Model file for the job. Use its own axes, mm. Coordinates: 2 decimals unless noted, no trailing zeros. Write each loop counter-clockwise with the first axis right and the second up, starting at its lowest first coordinate (ties: lowest second). Pieces come first, ordered by that corner, then holes.
Q1. Drill centre lines: probe 1 along Y at (x, z) = (6.5, 25); probe 2 along Z at (x, y) = (5, -4); probe 3 along Z at (x, y) = (12, -1.5). Where is each one in solid material? Low to high.
Q2. Band-saw the part on B-B, the plane z = 25. Write the cut outline in (x, y).
Q3. Pin check, flat tip, straight feed: P1, Ø10, axis at y = 0, z = 265, coming from the -X side. Stop position of the tip, or through.
Q4. Band-saw the part on A-A, the plane y = 0. Write the cut outline in (x, z).
Q5. Band-saw the part on C-C, the plane x = 9.5. Write the cut outline in (y, z).
Q6. Pull direction Z, two halves, no side cores. Call faces 1 (the flat face through (0, 0, 290)), 2 (the flat face through (15, 0, 143)), 3 (the cylindrical face through (-0.21, 1.652, 270.246)): released by +Z, released by -Z, zero draft, split by the parting line, or undercut.
from build123d import *

# Parameters (mm, degrees)
ESBO_O1_W                = 30
ESBO_O1_H                = 25
RESSALTO_EXTRUS_O2_DEPTH = 290
ESBO_O2_R                = 5.5
CORTE_EXTRUS_O1_DEPTH    = 290


with BuildPart() as part:
    # Esboço1 → Ressalto-extrusão2 (new body)
    with BuildSketch(Plane.XY):
        Rectangle(ESBO_O1_W, ESBO_O1_H)
    extrude(amount=RESSALTO_EXTRUS_O2_DEPTH)

    # Esboço2 → Corte-extrusão1 (cut)
    with BuildSketch(Plane.ZY.offset(15)):
        with Locations((25, 0)):
            Circle(ESBO_O2_R)
        with Locations((265, 0)):
            Circle(ESBO_O2_R)
    extrude(amount=-CORTE_EXTRUS_O1_DEPTH, mode=Mode.SUBTRACT)


solid = part.part
Answer sheet:
1. probe 1: y = -12.5 to -5.5, 5.5 to 12.5
1. probe 2: z = 0 to 21.23, 28.77 to 261.23, 268.77 to 290
1. probe 3: z = 0 to 19.71, 30.29 to 259.71, 270.29 to 290
2. outline: (-15, -12.5) - (15, -12.5) - (15, -5.5) - (-15, -5.5) - close; (-15, 5.5) - (15, 5.5) - (15, 12.5) - (-15, 12.5) - close
3. P1: passes through
4. outline: (-15, 0) - (15, 0) - (15, 19.5) - (-15, 19.5) - close; (-15, 30.5) - (15, 30.5) - (15, 259.5) - (-15, 259.5) - close; (-15, 270.5) - (15, 270.5) - (15, 290) - (-15, 290) - close
5. outline: (-12.5, 0) - (12.5, 0) - (12.5, 290) - (-12.5, 290) - close; hole circle Ø11 at (0, 25); hole circle Ø11 at (0, 265)
6. face 1: released by +Z
6. face 2: zero draft
6. face 3: undercut
